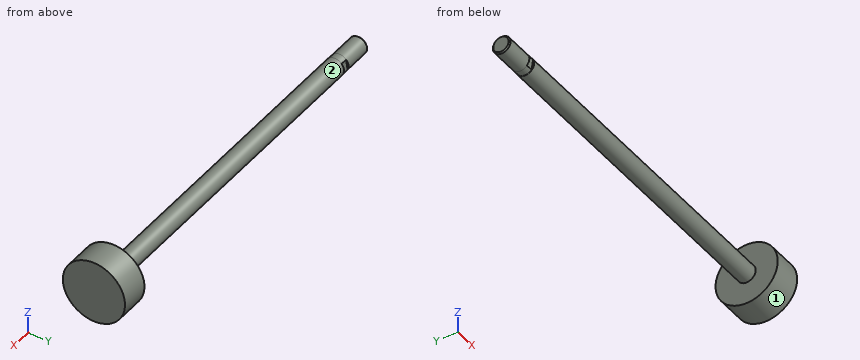
```python
from build123d import *

# Parameters (mm, degrees)
SKETCH1_W           = 12.7
SKETCH1_H           = 3.86334
BOSS_EXTRUDE1_DEPTH = 3.048
SKETCH3_R           = 3.9624
BOSS_EXTRUDE2_DEPTH = 144.526
SKETCH4_R           = 13.49375
BOSS_EXTRUDE3_DEPTH = 12.7
CHAMFER1_SIZE       = 0.53594


with BuildPart() as part:
    # Sketch1 → Revolve1 (revolve)
    with BuildSketch(Plane.XY):
        with Locations((739.199890203, 1.93167)):
            Rectangle(SKETCH1_W, SKETCH1_H)
    revolve(axis=Axis((732.849890203, 0, 0), (1, 0, 0)))

    # Sketch2 → Boss-Extrude1 (add)
    with BuildSketch(Plane(origin=(745.549890203, 0, 0), x_dir=(0, 0, -1), z_dir=(1, 0, 0))):
        with BuildLine():
            Line((2.623507611, -2.835948478), (-1.73539242, -3.451638611))
            ThreePointArc((-1.73539242, -3.451638611), (-3.825367985, -0.540329282), (-2.623507611, 2.835948478))
            Line((-2.623507611, 2.835948478), (1.73539242, 3.451638611))
            ThreePointArc((1.73539242, 3.451638611), (3.825367985, 0.540329282), (2.623507611, -2.835948478))
        make_face()
    extrude(amount=BOSS_EXTRUDE1_DEPTH)

    # Sketch3 → Boss-Extrude2 (add)
    with BuildSketch(Plane(origin=(748.597890203, 0, 0), x_dir=(0, -1, 0), z_dir=(-1, 0, 0))):
        Circle(SKETCH3_R)
    extrude(amount=-BOSS_EXTRUDE2_DEPTH)

    # Sketch4 → Boss-Extrude3 (add)
    with BuildSketch(Plane(origin=(893.123890203, 0, 0), x_dir=(0, -1, 0), z_dir=(-1, 0, 0))):
        Circle(SKETCH4_R)
    extrude(amount=-BOSS_EXTRUDE3_DEPTH)

    # Chamfer1
    chamfer1_edges = [part.edges().sort_by_distance(p)[0] for p in [
        (732.849890203, -3.86334, 0),
    ]]
    chamfer(chamfer1_edges, length=CHAMFER1_SIZE)


solid = part.part
```
Check sheet for the modelled part. Datum: model origin and axes. Units: mm. Face numbers are marked on the shaded views. A direction names the side the tool comes from. Round coordinates to 2 decimals unless told otherwise and drop trailing zeros. Order: outer loops, then holes, each group sorted by start corner. A loop starts at its lowest first (then second) coordinate and runs counter-clockwise, first axis right, second up.
1) Section check C-C (x = 773). Record the boundary of the cut face in (y, z), and give its area (3 significant figures).
2) Section check A-A (y = 0). Record the boundary of the cut face in (x, z), and give its area (3 significant figures).
3) Section check B-B (z = 0). Record the boundary of the cut face in (x, y).
4) Scan lines: line 1 (X direction, y = -5.25, z = -8.75); line 2 (Y direction, x = 887.5, z = -1); line 3 (Y direction, x = 843.5, z = 0.25). Record each from-to range of solid material in increasing order.
5) Tool access check on the marked faces 1 and 2. Record the directions out of +Z, -Z, +X, -X, +Y, -Y that give a thin tool (end or side, any length) a straight path to the whole face; none if there is none.
6) Section check D-D (y = -8). Record the boundary of the cut face in (x, z).
7) Go/stop test with flat-tipped pins: pin 1 Ø10 at (x, y) = (829, -6.5) entering from -Z; pin 2 Ø8 at (x, z) = (855, -6.5) entering from -Y; pin 3 Ø12 at (x, y) = (888.5, -9) entering from +Z. Record where each tip stops, or that it passes through.
Result:
1. outline: circle Ø7.92 at (0, 0)
1. area: 49.3 mm2
2. outline: (732.85, -3.33) - (733.39, -3.86) - (748.6, -3.86) - (748.6, -3.96) - (893.12, -3.96) - (893.12, -13.49) - (905.82, -13.49) - (905.82, 13.49) - (893.12, 13.49) - (893.12, 3.96) - (748.6, 3.96) - (748.6, 3.86) - (733.39, 3.86) - (732.85, 3.33) - close
2. area: 1,610 mm2
3. outline: (732.85, -3.33) - (733.39, -3.86) - (745.55, -3.86) - (745.55, -3.21) - (748.6, -3.21) - (748.6, -3.96) - (893.12, -3.96) - (893.12, -13.49) - (905.82, -13.49) - (905.82, 13.49) - (893.12, 13.49) - (893.12, 3.96) - (748.6, 3.96) - (748.6, 3.21) - (745.55, 3.21) - (745.55, 3.86) - (733.39, 3.86) - (732.85, 3.33) - close
4. line 1: x = 893.12 to 905.82
4. line 2: y = -3.83 to 3.83
4. line 3: y = -3.95 to 3.95
5. face 1: +X, -X
5. face 2: -X
6. outline: (893.12, -10.87) - (905.82, -10.87) - (905.82, 10.87) - (893.12, 10.87) - close
7. pin 1: stops at z = -3.67
7. pin 2: stops at y = -3.07
7. pin 3: stops at z = 12.46
